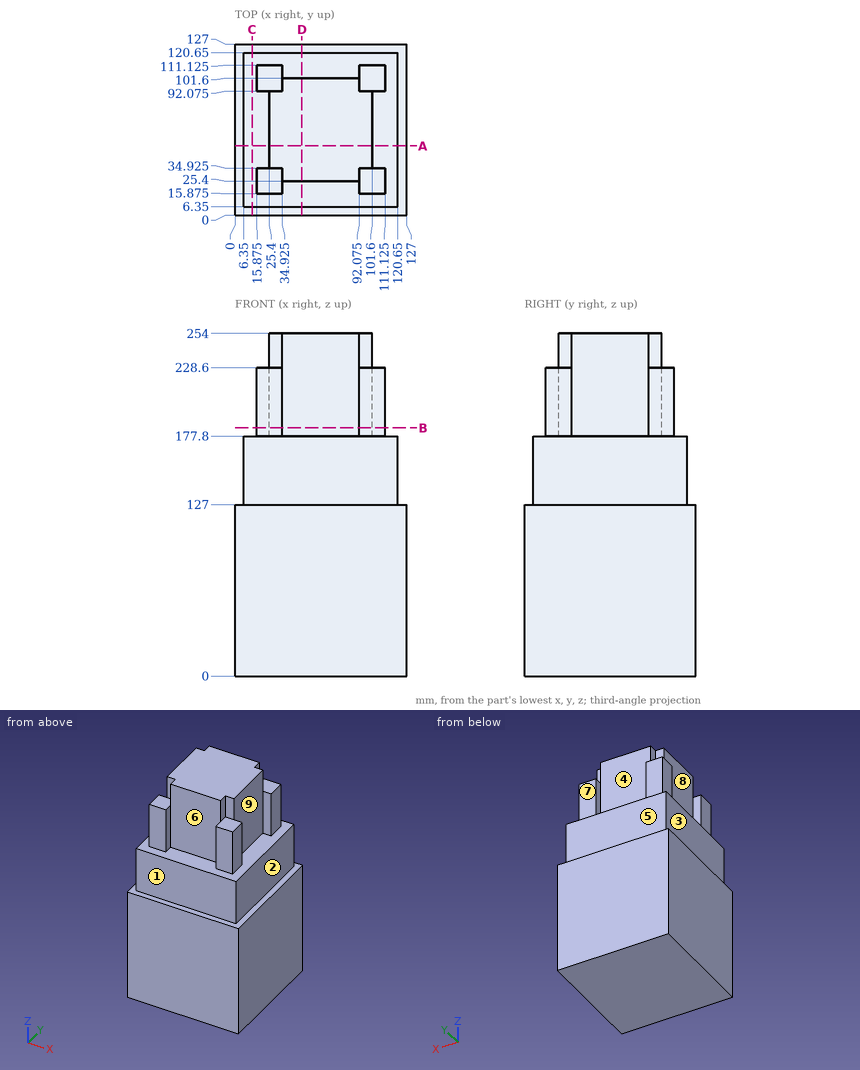
Drawing for the job (mm, zero at the part's lowest x, y, z). A direction names the side the tool comes from. Coordinates: 2 decimals unless noted, no trailing zeros. Order: outer loops, then holes, each group sorted by start corner. A loop starts at its lowest first (then second) coordinate and runs counter-clockwise, first axis right, second up. Notation, with made-up numbers: (5.5, 23.25) -> (17.5, 23.25) arc R15 ccw to (17.5, 35.25) -> close; hole circle Ø8 at (46, 39.5). An arc over 180 degrees is marked (long way). Return JSON: item names as keys, results as strings.
Item 1: 3-axis set-ups, long thin cutter, end or side, ignore diameter. For the marked faces 1, 2, 3, 4 and 5: which of +Z, -Z, +X, -X, +Y, -Y reach the whole face in a straight line?
Model answer:
{"face 1": "+Z, +X, -X, -Y", "face 2": "+Z, +X, +Y, -Y", "face 3": "+Z, -X, +Y, -Y", "face 4": "+Z, +Y", "face 5": "+Z, +X, -X, +Y"}
Item 2: Wall check: line 1 along Y through (x, z) = (20, 212) (3 decimals); line 2 along Y through (x, z) = (19.5, 164.5); line 3 along Z through (x, y) = (14, 54). Give the ranges that are in metal, low to high. Write a range as from..to.
Model answer:
{"line 1": "y = 15.875..34.925, 92.075..111.125", "line 2": "y = 6.35..120.65", "line 3": "z = 0..177.8"}
Item 3: Pin check, flat tips, straight feed: P1, Ø7.5, axis at y = 28, z = 240.5, coming from the +X side (3 decimals); P2, Ø7.5, axis at x = 20.5, z = 193.5, coming from the -Y side (3 decimals); P3, Ø12, axis at x = 68, z = 160, coming from the -Y side. Stop position of each tip, or through.
Model answer:
{"P1": "stops at x = 92.075", "P2": "stops at y = 15.875", "P3": "stops at y = 6.35"}
Item 4: Slice it at C-C (x = 12.5). Write the cut outline in (y, z), then the cut area to 3 significant figures.
Model answer:
{"outline": "(0, 0) -> (127, 0) -> (127, 127) -> (120.65, 127) -> (120.65, 177.8) -> (6.35, 177.8) -> (6.35, 127) -> (0, 127) -> close", "area": "21,900 mm²"}
Item 5: Slice it at B-B (z = 184). Write the cut outline in (x, y) (3 decimals), then the cut area to 3 significant figures.
Model answer:
{"outline": "(15.875, 15.875) -> (34.925, 15.875) -> (34.925, 25.4) -> (92.075, 25.4) -> (92.075, 15.875) -> (111.125, 15.875) -> (111.125, 34.925) -> (101.6, 34.925) -> (101.6, 92.075) -> (111.125, 92.075) -> (111.125, 111.125) -> (92.075, 111.125) -> (92.075, 101.6) -> (34.925, 101.6) -> (34.925, 111.125) -> (15.875, 111.125) -> (15.875, 92.075) -> (25.4, 92.075) -> (25.4, 34.925) -> (15.875, 34.925) -> close", "area": "6,900 mm²"}
Item 6: Slice it at A-A (y = 51.5). Write the cut outline in (x, z), then the cut area to 3 significant figures.
Model answer:
{"outline": "(0, 0) -> (127, 0) -> (127, 127) -> (120.65, 127) -> (120.65, 177.8) -> (101.6, 177.8) -> (101.6, 254) -> (25.4, 254) -> (25.4, 177.8) -> (6.35, 177.8) -> (6.35, 127) -> (0, 127) -> close", "area": "27,700 mm²"}
Item 7: Mould opens along Y. For the marked faces 6, 7, 8 and 9 say: pulls with the +Y half, pulls with the -Y half, needs draft (parallel to the pull), parting line crosses it, or undercut.
Model answer:
{"face 6": "pulls with the -Y half", "face 7": "pulls with the +Y half", "face 8": "undercut", "face 9": "undercut"}
